from build123d import *

# Parameters (mm, degrees)
F1_DEPTH = 31.75
F2_DEPTH = 25.4
F3_DEPTH = 12.7
F5_DEPTH = 6.35
F6_R     = 3.175
F7_DEPTH = 6.35


with BuildPart() as f1:
    # F0 (on Front) → F1 (new body)
    with BuildSketch(Plane.XZ):
        Polygon((-42.646856, 0), (-55.346856, 0), (-55.346856, -6.35), (-4.546856, -6.35), (-4.546856, 0), (-17.246856, 0), align=None)
    extrude(amount=F1_DEPTH)



with BuildPart() as f2:
    # F0 (on Front) → F2 (new body)
    with BuildSketch(Plane.XZ):
        with BuildLine():
            ThreePointArc((-17.246856, 38.1), (-20.9666, 47.080256), (-29.946856, 50.8))
            ThreePointArc((-29.946856, 50.8), (-38.927112, 47.080256), (-42.646856, 38.1))
            ThreePointArc((-42.646856, 38.1), (-29.946856, 25.4), (-17.246856, 38.1))
        make_face()
        with BuildLine():
            ThreePointArc((-23.596856, 38.1), (-34.436984, 33.609872), (-29.946856, 44.45))
            ThreePointArc((-29.946856, 44.45), (-25.456728, 42.590128), (-23.596856, 38.1))
        make_face(mode=Mode.SUBTRACT)
    extrude(amount=F2_DEPTH)


with BuildPart() as f1_1:
    add(f1.part)

    add(f2.part)  # F3 merges F2
    # F0 (on Front) → F3 (join)
    with BuildSketch(Plane.XZ):
        with BuildLine():
            ThreePointArc((-42.646856, 12.7), (-46.3666, 3.719744), (-55.346856, 0))
            Line((-55.346856, 0), (-42.646856, 0))
            Line((-42.646856, 0), (-17.246856, 0))
            Line((-17.246856, 0), (-4.546856, 0))
            ThreePointArc((-4.546856, 0), (-13.527112, 3.719744), (-17.246856, 12.7))
            Line((-17.246856, 12.7), (-17.246856, 38.1))
            ThreePointArc((-17.246856, 38.1), (-29.946856, 25.4), (-42.646856, 38.1))
            Line((-42.646856, 38.1), (-42.646856, 12.7))
        make_face()
    extrude(amount=F3_DEPTH)

    # F4 (on face) → F5 (cut)
    with BuildSketch(Plane.XY):
        with BuildLine():
            ThreePointArc((-42.646856, -31.75), (-51.627112, -28.030256), (-55.346856, -19.05))
            Line((-55.346856, -19.05), (-55.346856, -31.75))
            Line((-55.346856, -31.75), (-42.646856, -31.75))
        make_face()
        with BuildLine():
            Line((-4.546856, -31.75), (-4.546856, -19.05))
            ThreePointArc((-4.546856, -19.05), (-8.2666, -28.030256), (-17.246856, -31.75))
            Line((-17.246856, -31.75), (-4.546856, -31.75))
        make_face()
    extrude(amount=-F5_DEPTH, mode=Mode.SUBTRACT)

    # F6 (on face) → F7 (cut)
    with BuildSketch(Plane.XY):
        with Locations((-45.552474, -22.190144)):
            Circle(F6_R)
        with Locations((-14.071856, -22.20941)):
            Circle(F6_R)
    extrude(amount=-F7_DEPTH, mode=Mode.SUBTRACT)


solid = f1_1.part
Work out the finished part from the listing and answer in its coordinate system (mm). A direction names the side the tool comes from. Give positions to 0.01 mm unless a question says otherwise; leave off trailing zeros. Loops run counter-clockwise (first coordinate to the right, second up) from the corner with the lowest first, then second, coordinate; pieces in that order, holes last. Notation, with made-up numbers: (3, 34) - (23, 34) arc R17 ccw to (23, 40) - close; hole circle Ø2 at (21.5, 88.5). An arc over 180 degrees is marked (long way). Answer in a Markdown table with one row per item.
(1) Flat-ended cylindrical pins translate along their axes: pin 1 Ø10 at (x, z) = (-43.5, 43) entering from -Y; pin 2 Ø1.5 at (x, z) = (-20.5, 4) entering from +Y; pin 3 Ø10 at (y, z) = (-4.5, 22) entering from +X; pin 4 Ø4 at (x, y) = (-13, -9) entering from +Z. Find the tip coordinate at first contact, or state that the pin passes through.
Results list:
| item | result |
|---|---|
| pin 1 | stops at y = -25.4 |
| pin 2 | stops at y = 0 |
| pin 3 | stops at x = -17.25 |
| pin 4 | stops at z = 5.49 |
(2) Section C-C (x = -35) is taken. Give the vertices of the cut face in (y, z).
Results list:
| item | result |
|---|---|
| outline | (-31.75, -6.35) - (0, -6.35) - (0, 34.25) - (-25.4, 34.25) - (-25.4, 26.45) - (-12.7, 26.45) - (-12.7, 0) - (-31.75, 0) - close; (-25.4, 41.95) - (0, 41.95) - (0, 49.75) - (-25.4, 49.75) - close |
(3) For a pull along Z with two mould halves and no side action, classify faces 1 (the face through (-11.14, -23.43, -3.13)), 2 (the face through (-30, -12.7, 15)), 3 (the face through (-30, -22, 0)), 4 (the face through (-30, -16, -6.35)) as pulls with the +Z half, pulls with the -Z half, needs draft (parallel to the pull), parting line crosses it, or undercut.
Results list:
| item | result |
|---|---|
| face 1 | needs draft |
| face 2 | undercut |
| face 3 | undercut |
| face 4 | pulls with the -Z half |
(4) Section A-A (y = -11) is taken. Give the vertices of the cut face in (x, z).
Results list:
| item | result |
|---|---|
| outline | (-55.35, -6.35) - (-4.55, -6.35) - (-4.55, 0) arc R12.7 cw to (-17.25, 12.7) - (-17.25, 38.1) arc R12.7 ccw to (-42.65, 38.1) - (-42.65, 12.7) arc R12.7 cw to (-55.35, 0) - close; hole circle Ø12.7 at (-29.95, 38.1) |
(5) Consider L1, parallel to X at y = -17, z = 38; L2, parallel to Y at x = -23, z = 27; L3, parallel to X at y = -2, z = 22. Determine where each line is inside the solid, lowest interval first. Write a range as [from, to].
Results list:
| item | result |
|---|---|
| L1 | x = [-42.65, -36.3], [-23.6, -17.25] |
| L2 | y = [-12.7, 0] |
| L3 | x = [-42.65, -17.25] |
(6) Section B-B (x = -15) is taken. Give the vertices of the cut face in (y, z).
Results list:
| item | result |
|---|---|
| outline | (-31.55, -6.35) - (-25.25, -6.35) - (-25.25, 0) - (-31.55, 0) - close; (-19.17, -6.35) - (0, -6.35) - (0, 5.49) - (-12.7, 5.49) - (-12.7, 0) - (-19.17, 0) - close |
(7) Section D-D (z = 30) is taken. Give the vertices of the cut face in (x, y), and give its area (3 significant figures).
Results list:
| item | result |
|---|---|
| outline | (-42.65, -12.7) - (-39.73, -12.7) - (-39.73, -25.4) - (-20.17, -25.4) - (-20.17, -12.7) - (-17.25, -12.7) - (-17.25, 0) - (-42.65, 0) - close |
| area | 571 mm² |
(8) A tool of negligible diameter and unlimited length cuts with its end or side. For faces 5 (the face through (-42.647, -6, 26)), 6 (the face through (-36, -25.4, 35)), 7 (the face through (-48.724, -22.051, -3.131)), 8 (the face through (-17.247, -6, 25)), 9 (the face through (-51.528, -28.128, -3.131)), from which of +Z, -Z, +X, -X, +Y, -Y can it reach the whole face along a straight path? Write none if from no direction.
Results list:
| item | result |
|---|---|
| face 5 | +Z, -X, +Y, -Y |
| face 6 | +Z, +X, -X, -Y |
| face 7 | -Z |
| face 8 | +Z, +X, +Y, -Y |
| face 9 | +Z, -Z, -X, -Y |
